Here's how the part is built. I have some questions about the finished solid (model axes, mm). A direction names the side the tool comes from. Coordinates: 2 decimals unless noted, no trailing zeros. Write each loop counter-clockwise with the first axis right and the second up, starting at its lowest first coordinate (ties: lowest second). Pieces come first, ordered by that corner, then holes.
from build123d import *

# Parameters (mm, degrees)
CUT_EXTRUDE1_DEPTH = 7.562178
FILLET1_R          = 0.5


with BuildPart() as part:
    # Sketch1 → Revolve1 (revolve)
    with BuildSketch(Plane.XY, mode=Mode.PRIVATE) as revolve1_sk:
        with BuildLine():
            Line((6.633974596215569, -1.2e-16), (8.999999999999998, -4.52e-15))
            Line((8.999999999999998, -4.52e-15), (8.999999999999998, 1.4999999999999956))
            Line((8.999999999999998, 1.4999999999999956), (7.5, 1.5))
            Line((7.5, 1.5), (4, 7.562177826491056))
            ThreePointArc((4, 7.562177826491056), (3.99763327378791, 8.432186632808357), (4.294453456567456, 9.249999999999998))
            ThreePointArc((4.294453456567456, 9.249999999999998), (5.662653405718452, 10.973935293777526), (7.4723600696108665, 12.226487004746774))
            Line((7.4723600696108665, 12.226487004746774), (6.808903286542892, 13.57178440569613))
            ThreePointArc((6.808903286542892, 13.57178440569613), (4.6372552898719945, 12.068722352533033), (2.995415350890799, 10))
            ThreePointArc((2.995415350890799, 10), (2.4999999999999996, 8.15108473962598), (2.995415350890799, 6.302169479251957))
            Line((2.995415350890799, 6.302169479251957), (6.633974596215569, -1.2e-16))
        make_face()
    revolve(revolve1_sk.sketch.rotate(Axis((0, 0, 0), (0, 1, 0)), 90), axis=Axis((0, 0, 0), (0, 1, 0)))

    # Sketch2 → Cut-Extrude1 (cut)
    with BuildSketch(Plane(origin=(0, 0, 0), x_dir=(1, 0, 0), z_dir=(0, 1, 0))):
        with BuildLine():
            Line((-3.749999941549397, 6.495190562129763), (-1.999999941549405, 3.4641016488842244))
            ThreePointArc((-1.999999941549405, 3.4641016488842244), (2.4e-16, 4.0000000000000036), (1.999999941549405, 3.4641016488842244))
            Line((1.999999941549405, 3.4641016488842244), (3.749999941549397, 6.495190562129763))
            ThreePointArc((3.749999941549397, 6.495190562129763), (4.6e-16, 7.500000000000002), (-3.749999941549397, 6.495190562129763))
        make_face()
        with BuildLine():
            Line((6.495190562129763, 3.7499999415493974), (3.4641016488842244, 1.999999941549405))
            ThreePointArc((3.4641016488842244, 1.999999941549405), (4.0000000000000036, 0), (3.4641016488842244, -1.999999941549405))
            Line((3.4641016488842244, -1.999999941549405), (6.495190562129763, -3.7499999415493965))
            ThreePointArc((6.495190562129763, -3.7499999415493965), (7.500000000000002, 0), (6.495190562129763, 3.7499999415493974))
        make_face()
        with BuildLine():
            Line((3.749999941549398, -6.495190562129762), (1.9999999415494054, -3.464101648884224))
            ThreePointArc((1.9999999415494054, -3.464101648884224), (2.4e-16, -4.0000000000000036), (-1.9999999415494045, -3.464101648884225))
            Line((-1.9999999415494045, -3.464101648884225), (-3.749999941549396, -6.495190562129764))
            ThreePointArc((-3.749999941549396, -6.495190562129764), (2.12e-15, -7.500000000000003), (3.749999941549398, -6.495190562129762))
        make_face()
        with BuildLine():
            Line((-6.495190562129762, -3.7499999415493983), (-3.464101648884224, -1.9999999415494054))
            ThreePointArc((-3.464101648884224, -1.9999999415494054), (-4.0000000000000036, 4.9e-16), (-3.464101648884225, 1.9999999415494045))
            Line((-3.464101648884225, 1.9999999415494045), (-6.495190562129764, 3.7499999415493956))
            ThreePointArc((-6.495190562129764, 3.7499999415493956), (-7.500000000000002, -2.41e-15), (-6.495190562129762, -3.7499999415493983))
        make_face()
    extrude(amount=CUT_EXTRUDE1_DEPTH, mode=Mode.SUBTRACT)

    # Fillet1
    # the kernel refuses this fillet: 0.5 mm, written as the material it adds along each edge
    with BuildSketch(Plane(origin=(0, 1.5, 0), x_dir=(0.8660254082839624, 0, -0.49999999220659597), z_dir=(0.49999999220659597, 0, 0.8660254082839624))) as fillet1_piece_1:
        with BuildLine():
            CenterArc((7.499999999999999 + FILLET1_R * 0.57735026919, FILLET1_R), FILLET1_R, 209.99999999999957, 60.000000000000455)
            Line((7.499999999999999 - FILLET1_R * 0.288675134595, FILLET1_R * 0.5), (7.499999999999999, 0))
            Line((7.499999999999999, 0), (7.499999999999999 + FILLET1_R * 0.57735026919, -4.44e-15))
        make_face()
    revolve(axis=Axis((0, 1.5, 0), (0, 1, 0)), revolution_arc=30.000001031215383)
    with BuildSketch(Plane(origin=(0, 1.5, 0), x_dir=(0.4999999922066019, 0, 0.8660254082839591), z_dir=(-0.8660254082839591, 0, 0.4999999922066019))) as fillet1_piece_2:
        with BuildLine():
            CenterArc((7.5 + FILLET1_R * 0.57735026919, FILLET1_R), FILLET1_R, 209.99999999999957, 60.000000000000455)
            Line((7.5 - FILLET1_R * 0.288675134595, FILLET1_R * 0.5), (7.5, 0))
            Line((7.5, 0), (7.5 + FILLET1_R * 0.57735026919, -4.44e-15))
        make_face()
    revolve(axis=Axis((0, 1.5, 0), (0, 1, 0)), revolution_arc=30.000001031214644)
    with BuildSketch(Plane(origin=(0, 1.5, 0), x_dir=(-0.8660254082839636, 0, 0.49999999220659425), z_dir=(-0.49999999220659425, 0, -0.8660254082839636))) as fillet1_piece_3:
        with BuildLine():
            CenterArc((7.5 + FILLET1_R * 0.57735026919, FILLET1_R), FILLET1_R, 209.99999999999963, 60.00000000000034)
            Line((7.5 - FILLET1_R * 0.288675134595, FILLET1_R * 0.5), (7.5, 0))
            Line((7.5, 0), (7.5 + FILLET1_R * 0.57735026919, -4.44e-15))
        make_face()
    revolve(axis=Axis((0, 1.5, 0), (0, 1, 0)), revolution_arc=30.000001031214545)
    with BuildSketch(Plane(origin=(0, 1.5, 0), x_dir=(-0.49999999220658903, 0, -0.8660254082839666), z_dir=(0.8660254082839666, 0, -0.49999999220658903))) as fillet1_piece_4:
        with BuildLine():
            CenterArc((7.499999999999999 + FILLET1_R * 0.57735026919, FILLET1_R), FILLET1_R, 210.00000000000003, 59.99999999999987)
            Line((7.499999999999999 + FILLET1_R * 0.57735026919, 4.4e-16), (7.499999999999999, 0))
            Line((7.499999999999999, 0), (7.499999999999999 - FILLET1_R * 0.288675134595, FILLET1_R * 0.5))
        make_face()
    revolve(axis=Axis((0, 1.5, 0), (0, 1, 0)), revolution_arc=30.00000103121539)
    # the kernel refuses this fillet: 0.5 mm, written as the material it takes off along each edge
    with BuildSketch(Plane(origin=(0, -1.2e-16, 0), x_dir=(0.9151940117210042, 0, -0.40301354928837607), z_dir=(0.40301354928837607, 0, 0.9151940117210042))) as fillet1_2_piece_1:
        with BuildLine():
            CenterArc((6.633974596215569 + FILLET1_R * 0.57735026919, FILLET1_R), FILLET1_R, 210.00000000000003, 59.99999999999987)
            Line((6.633974596215569 + FILLET1_R * 0.57735026919, -1.27e-15), (6.633974596215569, 1.2e-16))
            Line((6.633974596215569, 1.2e-16), (6.633974596215569 - FILLET1_R * 0.288675134595, FILLET1_R * 0.5))
        make_face()
    revolve(axis=Axis((0, -1.2e-16, 0), (0, 1, 0)), revolution_arc=42.466588641203785, mode=Mode.SUBTRACT)
    with BuildSketch(Plane(origin=(0, -1.2e-16, 0), x_dir=(0.40301354928837646, 0, 0.915194011721004), z_dir=(-0.915194011721004, 0, 0.40301354928837646))) as fillet1_2_piece_2:
        with BuildLine():
            CenterArc((6.633974596215568 + FILLET1_R * 0.57735026919, FILLET1_R), FILLET1_R, 210.00000000000006, 59.999999999999844)
            Line((6.633974596215568 + FILLET1_R * 0.57735026919, -3.3e-16), (6.633974596215568, 1.2e-16))
            Line((6.633974596215568, 1.2e-16), (6.633974596215568 - FILLET1_R * 0.288675134595, FILLET1_R * 0.5))
        make_face()
    revolve(axis=Axis((0, -1.2e-16, 0), (0, 1, 0)), revolution_arc=42.466588641203685, mode=Mode.SUBTRACT)
    with BuildSketch(Plane(origin=(0, -1.2e-16, 0), x_dir=(-0.915194011721004, 0, 0.4030135492883765), z_dir=(-0.4030135492883765, 0, -0.915194011721004))) as fillet1_2_piece_3:
        with BuildLine():
            CenterArc((6.633974596215569 + FILLET1_R * 0.57735026919, FILLET1_R), FILLET1_R, 210.0000000000001, 59.999999999999886)
            Line((6.633974596215569 + FILLET1_R * 0.57735026919, -1.21e-15), (6.633974596215569, 1.2e-16))
            Line((6.633974596215569, 1.2e-16), (6.633974596215569 - FILLET1_R * 0.288675134595, FILLET1_R * 0.5))
        make_face()
    revolve(axis=Axis((0, -1.2e-16, 0), (0, 1, 0)), revolution_arc=42.466588641203685, mode=Mode.SUBTRACT)
    with BuildSketch(Plane(origin=(0, -1.2e-16, 0), x_dir=(-0.40301354928837607, 0, -0.9151940117210042), z_dir=(0.9151940117210042, 0, -0.40301354928837607))) as fillet1_2_piece_4:
        with BuildLine():
            CenterArc((6.63397459621557 + FILLET1_R * 0.57735026919, FILLET1_R), FILLET1_R, 210.00000000000006, 59.99999999999994)
            Line((6.63397459621557 + FILLET1_R * 0.57735026919, -1.21e-15), (6.63397459621557, 1.2e-16))
            Line((6.63397459621557, 1.2e-16), (6.63397459621557 - FILLET1_R * 0.288675134595, FILLET1_R * 0.5))
        make_face()
    revolve(axis=Axis((0, -1.2e-16, 0), (0, 1, 0)), revolution_arc=42.46658864120374, mode=Mode.SUBTRACT)
    with BuildSketch(Plane(origin=(0, 13.571784405696132, 0), x_dir=(1.1e-16, 0, -1), z_dir=(1, 0, 1.1e-16))) as fillet1_2_piece_5:
        with BuildLine():
            CenterArc((6.5881331953149616, -0.6827853473273997), FILLET1_R, 26.25101140415418, 93.3722866833914)
            Line((7.036565662297915, -0.46163308630440625), (6.808903286542892, 0))
            ThreePointArc((6.808903286542892, 0), (6.573118661901752, -0.12062636424792572), (6.3409855018069745, -0.2481383438939453))
        make_face()
    revolve(axis=Axis((0, 13.571784405696132, 0), (0, 1, 0)), mode=Mode.SUBTRACT)
    with BuildSketch(Plane(origin=(0, 12.226487004746774, 0), x_dir=(1.1e-16, 0, -1), z_dir=(1, 0, 1.1e-16))) as fillet1_2_piece_6:
        with BuildLine():
            CenterArc((6.809693112007429, 0.21325297950030375), FILLET1_R, 299.8343331025833, 86.41667830167688)
            Line((7.258125578989974, 0.43440524052412677), (7.4723600696108665, 0))
            ThreePointArc((7.4723600696108665, 0), (7.263676285711675, -0.10700426181869638), (7.058440041566387, -0.22048076951513984))
        make_face()
    revolve(axis=Axis((0, 12.226487004746774, 0), (0, 1, 0)), mode=Mode.SUBTRACT)


solid = part.part
1. On a 3-axis mill with a long thin cutter (end or side, diameter ignored), from which of +Z, -Z, +X, -X, +Y, -Y can I reach the whole of each face in a straight line? I mean faces 4 (the face through (0, 6, 4)), 5 (the face through (-3.984, 4.697, -4.013)), 6 (the face through (-4, 6, 0)), 7 (the face through (2, 1.5, 7.4)). Say none if no direction works.
2. I want a section at A-A (y = 2). List the corners of the cut face in (x, z) for me, then the cut area to 3 significant figures.
3. If I drill on line 1 (X direction, y = 3.75, z = 3.25); line 2 (Y direction, x = -2.25, z = 3.5); line 3 (Y direction, x = 2, z = 7.5), over which ranges is the centre line in solid material (lowest first)?
4. I want a section at D-D (y = 5). List the corners of the cut face in (x, z) for me, then the cut area to 3 significant figures.
5. For pin 1 Ø8 at (y, z) = (10, -5.5) entering from -X; pin 2 Ø1.5 at (y, z) = (10.5, -3.5) entering from +X; pin 3 Ø6 at (x, z) = (-2.5, 1) entering from +Y, each with a flat end and sliding along its axis, tell me the tip position at first contact or that it passes through.
6. I want a section at B-B (x = 2.5). State how many separate pieces and enclosed holes the cut face has, then the cut area to 3 significant figures.
7. Thinking about a two-plate mould opening in Y: for faces 1 (the face through (0.1, 0.7, -7.5)), 2 (the face through (3.984, 4.697, 4.013)), 3 (the face through (-2.43, 5.25, 2.66)), which applies, pulls with the +Y half, pulls with the -Y half, needs draft (parallel to the pull), parting line crosses it, or undercut?
Response values:
1. face 4: +Z, -Y
1. face 5: -Z, -X
1. face 6: -X, -Y
1. face 7: +Y
2. outline: (-6.25, -3.61) arc R7.21 ccw to (-3.61, -6.25) - (-2.74, -4.75) arc R5.48 cw to (-4.75, -2.74) - close; (-6.25, 3.61) - (-4.75, 2.74) arc R5.48 cw to (-2.74, 4.75) - (-3.61, 6.25) arc R7.21 ccw to start; (2.74, -4.75) - (3.61, -6.25) arc R7.21 ccw to (6.25, -3.61) - (4.75, -2.74) arc R5.48 cw to start; (2.74, 4.75) arc R5.48 cw to (4.75, 2.74) - (6.25, 3.61) arc R7.21 ccw to (3.61, 6.25) - close
2. area: 23.0 mm2
3. line 1: x = -5.28 to -3.07, 3.07 to 5.28
3. line 2: y = 4.28 to 7.28, 8.98 to 11.59
3. line 3: y = 0 to 1.5
4. outline: (-4.75, -2.74) arc R5.48 ccw to (-2.74, -4.75) - (-2, -3.46) arc R4 ccw to (2, -3.46) - (2.74, -4.75) arc R5.48 ccw to (4.75, -2.74) - (3.46, -2) arc R4 ccw to (3.46, 2) - (4.75, 2.74) arc R5.48 ccw to (2.74, 4.75) - (2, 3.46) arc R4 ccw to (-2, 3.46) - (-2.74, 4.75) arc R5.48 ccw to (-4.75, 2.74) - (-3.46, 2) arc R4 ccw to (-3.46, -2) - close; hole circle Ø7.49 at (0, 0)
4. area: 20.8 mm2
5. pin 1: stops at x = -6.94
5. pin 2: stops at x = 4.96
5. pin 3: stops at y = 12.92
6. separate pieces: 4
6. enclosed holes: 0
6. area: 48.0 mm2
7. face 1: needs draft
7. face 2: undercut
7. face 3: pulls with the -Y half
